Autodesk Inventor part; units mm, degrees
ref_plane "YZ Plane" through (0, 0, 0) normal (1, 0, 0) x (0, 1, 0)
ref_plane "XZ Plane" through (0, 0, 0) normal (0, 1, 0) x (-1, 0, 0)
ref_plane "XY Plane" through (0, 0, 0) normal (0, 0, 1) x (1, 0, 0)
sketch "Sketch1" plane through (0, 0, 0) normal (0, 0, 1) x (1, 0, 0)
  line L0 (-79.767, 50.3169) -> (-34.607, 50.3169)
  line L1 (-34.607, 50.3169) -> (-34.607, 40.9969)
  line L2 (-34.607, 40.9969) -> (-79.767, 40.9969)
  line L3 (-79.767, 40.9969) -> (-79.767, 50.3169)
  line L4 (-57.187, 40.9969) -> (-57.187, 50.3169)
  point P0 (0, 0)
  point P1 (-75.587, 45.6569)
  point P2 (-79.767, 45.6569)
  point P3 (-68.287, 45.6569)
  point P4 (-38.787, 45.6569)
  point P5 (-46.087, 45.6569)
  dimension "d0" = 45.16
  dimension "d1" = 9.32
  dimension "d2" = 4.18
  dimension "d3" = 7.3
extrude "Extrusion1" add sketch "Sketch1" along normal blind 5.99
hole "Hole1" at (-38.787, 45.6569, 0) at (-46.087, 45.6569, 0) at (-68.287, 45.6569, 0) at (-75.587, 45.6569, 0) direction (0, 0, 1) diameter 3 end through all
thread "Thread1"
thread "Thread2"
thread "Thread3"
thread "Thread4"
sketch "Sketch2" plane through (-79.767, 50.3169, 0) normal (0, 1, 0) x (1, 0, 0)
  line L0 (0, 0) -> (45.16, 0)
  line L1 (45.16, -5.99) -> (0, -5.99)
  arc A0 (23.0312, -3.4698) -> (23.0312, -2.5202) centre (25.2213, -2.995) ccw
  arc A1 (22.1288, -2.5202) -> (22.1288, -3.4698) centre (19.9387, -2.995) ccw
  arc A2 (22.1288, -3.4698) -> (23.0312, -3.4698) centre (22.58, -2.995) ccw
  arc A3 (23.0312, -2.5202) -> (22.1288, -2.5202) centre (22.58, -2.995) ccw
  point P0 (79.767, 0)
extrude "Extrusion2" cut sketch "Sketch2" against normal through all
properties part number "load_cell"
Work out the finished part from the listing and answer in its coordinate system (mm). A direction names the side the tool comes from. Round coordinates to 2 decimals unless told otherwise and drop trailing zeros. Order: outer loops, then holes, each group sorted by start corner. A loop starts at its lowest first (then second) coordinate and runs counter-clockwise, first axis right, second up. Notation, with made-up numbers: M 6.25,55.5 L 65.25,55.5 A11 cw 65.25,63.5 Z; hole C -7,7 d9. An arc over 180 degrees is marked long. Put each result on its own line as item: value. Start each with the question number.
Q1. A flat-ended cylindrical pin translates along its axis: pin 1 (3.5 mm diameter, centred on x = -59.83, z = 3, fed in from +Y). Find the tip coordinate at first contact, or state that the pin passes through.
Q2. Section B-B, the plane y = 45.75 is taken. Write down the section's boundary in (x, z) (3 decimals), and give its area (3 significant figures).
Q3. Straight lines are drawn through the part: L1, parallel to X at y = 45.75, z = 5.4; L2, parallel to X at y = 47.25, z = 1.8; L3, parallel to X at y = 49, z = 4. For each, find the intervals that lie inside material, in ascending order. Write a range as [from, to].
Q4. Section A-A, the plane z = 1.6 is taken. Write down the section's boundary in (x, y), and give its area (3 significant figures).
Q5. A tool of negligible diameter and unlimited length cuts with its end or side. For faces 4 (the flat face through (-58, 46, 0)), 5 (the cylindrical face through (-57.19, 45.72, 3.65)), from which of +Z, -Z, +X, -X, +Y, -Y can it reach the whole face along a straight path? Write none if from no direction.
Q6. Section C-C, the plane x = -38 is taken. Write down the section's boundary in (y, z).
Q7. For a pull along X with two mould halves and no side action, classify faces 1 (the cylindrical face through (-74.67, 44.47, 3.04)), 2 (the flat face through (-79.767, 46, 3)), 3 (the flat face through (-34.607, 46, 3)) as pulls with the +X half, pulls with the -X half, needs draft (parallel to the pull), parting line crosses it, or undercut.
Q8. Section D-D, the plane y = 48.5 is taken. Write down the section's boundary in (x, z) (3 decimals).
Findings below:
1. pin 1: passes through
2. outline: M -79.767,0 L -77.084,0 L -77.084,5.99 L -79.767,5.99 Z; M -74.09,0 L -69.784,0 L -69.784,5.99 L -74.09,5.99 Z; M -66.79,0 L -47.584,0 L -47.584,5.99 L -66.79,5.99 Z; M -44.59,0 L -40.284,0 L -40.284,5.99 L -44.59,5.99 Z; M -37.29,0 L -34.607,0 L -34.607,5.99 L -37.29,5.99 Z; hole M -57.638,2.52 A0.655 ccw -56.736,2.52 A2.241 ccw long -56.736,3.47 A0.655 ccw -57.638,3.47 A2.241 ccw long Z
2. area: 166 mm^2
3. L1: x = [-79.77, -77.08], [-74.09, -69.78], [-66.79, -47.58], [-44.59, -40.28], [-37.29, -34.61]
3. L2: x = [-79.77, -61.72], [-57.93, -56.44], [-52.65, -34.61]
3. L3: x = [-79.77, -61.83], [-57.83, -56.55], [-52.54, -34.61]
4. outline: M -79.77,41 L -61.58,41 L -61.58,50.32 L -79.77,50.32 Z; M -58.07,41 L -56.3,41 L -56.3,50.32 L -58.07,50.32 Z; M -52.79,41 L -34.61,41 L -34.61,50.32 L -52.79,50.32 Z; hole C -75.59,45.66 d3; hole C -68.29,45.66 d3; hole C -46.09,45.66 d3; hole C -38.79,45.66 d3
4. area: 327 mm^2
5. face 4: -Z, +X, -X, +Y, -Y
5. face 5: +Y, -Y
6. outline: M 41,0 L 44.38,0 L 44.38,5.99 L 41,5.99 Z; M 46.93,0 L 50.32,0 L 50.32,5.99 L 46.93,5.99 Z
7. face 1: undercut
7. face 2: pulls with the -X half
7. face 3: pulls with the +X half
8. outline: M -79.767,0 L -34.607,0 L -34.607,5.99 L -79.767,5.99 Z; hole M -57.638,2.52 A0.655 ccw -56.736,2.52 A2.241 ccw long -56.736,3.47 A0.655 ccw -57.638,3.47 A2.241 ccw long Z
